Work out the finished part from the listing and answer in its coordinate system (mm). Face numbers are marked on the shaded views. A direction names the side the tool comes from. Give positions to 0.01 mm unless a question says otherwise; leave off trailing zeros.
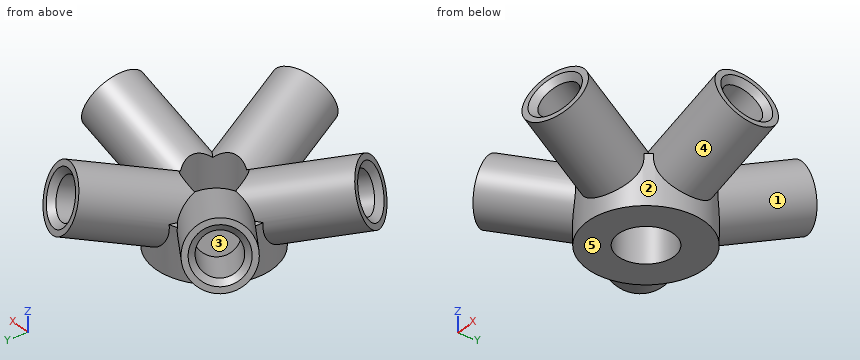
```python
from build123d import *

# Parameters (mm, degrees)
F3_COUNT = 5
F5_R     = 3.65
F6_DEPTH = 13.536313851
F7_SIZE  = 0.75


with BuildPart() as f2:
    # F1 (on Front) → F2 (revolve)
    with BuildSketch(Plane.XZ):
        Polygon((8.5060233307, 0.1325409275), (7.6729152797, 2.595452005), (7.6729152797, -1.7327594752), (18.364670155, 1.8838498077), (17.8840308948, 3.3047600447), align=None)
        Polygon((7.6729152797, 2.595452005), (0, 0), (1.3137473112, -3.8838213144), (7.6729152797, -1.7327594752), align=None)
    revolve(axis=Axis((8.5254614219, 0, 2.8838355611), (0.9472734913, 0, 0.3204261735)))

    # F3: F2 ×5 about axis
    f3_axis = Axis((0, 0, 20.6734314561), (0, 0, 1))


with BuildPart() as f2_1:
    add(f2.part)
    for i in range(1, F3_COUNT):
        add(f2.part.rotate(f3_axis, i * 360 / F3_COUNT))

    # F1 (on Front) → F4 (revolve)
    with BuildSketch(Plane.XZ):
        Polygon((1.3137473112, -3.8838213144), (0, 0), (0, -3.8838213144), align=None)
        Polygon((7.6729152797, 2.595452005), (0, 0), (1.3137473112, -3.8838213144), (7.6729152797, -1.7327594752), align=None)
        Polygon((7.6729152797, -1.7327594752), (1.3137473112, -3.8838213144), (7.6729152797, -3.8838213144), align=None)
        Polygon((0, 2.595452005), (0, 0), (7.6729152797, 2.595452005), align=None)
    revolve(axis=Axis((0, 0, 20.6734314561), (0, 0, 1)))

    # F5 (on face) → F6 (cut, through all)
    with BuildSketch(Plane(origin=(0, 0, -3.8838213144), x_dir=(1, 0, 0), z_dir=(0, 0, -1))):
        Circle(F5_R)
    extrude(amount=-F6_DEPTH, mode=Mode.SUBTRACT)

    # F7
    f7_edges = [f2_1.edges().sort_by_distance(p)[0] for p in [
        (-13.120488, -9.532592, 8.230582),
        (5.01158, -15.424058, 8.230582),
        (16.217815, 0, 8.230582),
        (5.01158, 15.424058, 8.230582),
        (-13.120488, 9.532592, 8.230582),
    ]]
    chamfer(f7_edges, length=F7_SIZE)


solid = f2_1.part
```
1. Straight lines are drawn through the part: probe 1 along X at (y, z) = (9.5, 5); probe 2 along Y at (x, z) = (0, 2); probe 3 along Y at (x, z) = (0, 1.75). For each, find the intervals that lie inside material, in ascending order.
Findings below:
probe 1: x = -8.8 to -6.45, -0.73 to 1.05, 5.45 to 7.23
probe 2: y = -11.99 to -3.65, 3.65 to 11.99
probe 3: y = -11.73 to -3.65, 3.65 to 11.73
2. The part is cut by section A-A (z = 7.5). State how many separate pieces and enclosed holes the cut face has, then the cut area to 3 significant figures.
Findings below:
separate pieces: 5
enclosed holes: 0
area: 151 mm2
3. Given P1, Ø1, axis at x = 9, z = 7.5, coming from the +Y side; P2, Ø2, axis at x = 4.5, z = 3.5, coming from the +Y side; P3, Ø2, axis at y = -3, z = 6.5, coming from the +X side; P4, Ø4.5, axis at x = 0, y = 0, coming from the +Z side, each flat-ended and moving along its own axis, determine where each tip first touches the part or whether it passes through.
Findings below:
P1: stops at y = 14.63
P2: stops at y = 17.75
P3: stops at x = 17.12
P4: passes through
4. Which of the six approach directions +Z, -Z, +X, -X, +Y, -Y give full straight-line access (tool end or side, diameter ignored) to the marked faces 1 and 2?
Findings below:
face 1: none
face 2: -Z
5. The mould has two halves that part along Z. Classify the marked faces 3, 4 and 5: pulls with the +Z half, pulls with the -Z half, needs draft (parallel to the pull), parting line crosses it, or undercut.
Findings below:
face 3: undercut
face 4: parting line crosses it
face 5: pulls with the -Z half
